Geometry check sheet. Reference: the model listing, model coordinates, mm. Face numbers are marked on the shaded views. Give positions to 0.01 mm unless a question says otherwise; leave off trailing zeros. Order: outer loops, then holes, each group sorted by start corner. A loop starts at its lowest first (then second) coordinate and runs counter-clockwise, first axis right, second up.
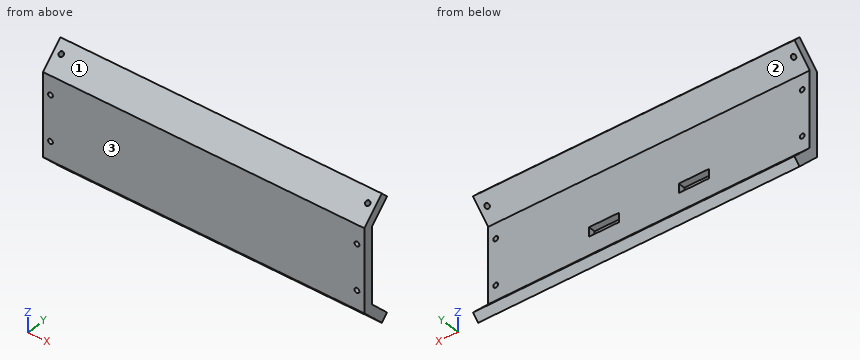
from build123d import *

# Parameters (mm, degrees)
MAIN_DEPTH                      = 107.5
F_4_0MM_DOWEL_HOLE2_D           = 3.2
F_4_0MM_DOWEL_HOLE2_ON_FACE_2_D = 3.2
F_4_0MM_DOWEL_HOLE2_ON_FACE_3_D = 3.2
F_4_0MM_DOWEL_HOLE2_ON_FACE_4_D = 3.2
SKETCH6_W                       = 20.125
SKETCH6_H                       = 6.125
SHELF_CUT_DEPTH                 = 116.995465651
SKETCH7_W                       = 20.125
SKETCH7_H                       = 6.125
BOSS_EXTRUDE2_DEPTH             = 1.4


with BuildPart() as part:
    # Sketch2 → Main (new, symmetric)
    with BuildSketch(Plane(origin=(0, 0, 0), x_dir=(0, 0, -1), z_dir=(1, 0, 0))):
        Polygon((-25, 0), (25, 0), (37.5, 12.5), (41.742640687, 8.257359313), (27.485281374, -6), (-27.485281374, -6), (-41.742640687, 8.257359313), (-37.5, 12.5), align=None)
    extrude(amount=MAIN_DEPTH, both=True)

    # Ø4.0mm Dowel Hole2 (through all)
    with Locations(Plane(origin=(-102.5, 7.071067812, -32.071067812), x_dir=(0, 0.707106781187, -0.707106781187), z_dir=(0, 0.707106781187, 0.707106781187))):
        with Locations((0, 0)):
            Hole(F_4_0MM_DOWEL_HOLE2_D / 2)

    # Ø4.0mm Dowel Hole2 on face 2 (through all)
    with Locations(Plane(origin=(-102.5, 0, -15), x_dir=(0, 0, 1), z_dir=(0, 1, 0))):
        with Locations((0, 0), (30, 0), (30, 205), (0, 205)):
            Hole(F_4_0MM_DOWEL_HOLE2_ON_FACE_2_D / 2)

    # Ø4.0mm Dowel Hole2 on face 3 (through all)
    with Locations(Plane(origin=(-102.5, 7.071067812, 32.071067812), x_dir=(0, -0.707106781187, -0.707106781187), z_dir=(0, 0.707106781187, -0.707106781187))):
        with Locations((0, 0), (0, -205)):
            Hole(F_4_0MM_DOWEL_HOLE2_ON_FACE_3_D / 2)

    # Ø4.0mm Dowel Hole2 on face 4 (through all)
    with Locations(Plane(origin=(102.5, 7.071067812, -32.071067812), x_dir=(0, 0.707106781187, -0.707106781187), z_dir=(0, 0.707106781187, 0.707106781187))):
        with Locations((0, 0)):
            Hole(F_4_0MM_DOWEL_HOLE2_ON_FACE_4_D / 2)

    # Sketch6 → Shelf cut (cut, through all)
    with BuildSketch(Plane(origin=(0, 0, 0), x_dir=(1, 0, 0), z_dir=(0, 1, 0))):
        with Locations((30, 10)):
            Rectangle(SKETCH6_W, SKETCH6_H)
        with Locations((-30, 10)):
            Rectangle(SKETCH6_W, SKETCH6_H)
    extrude(amount=-SHELF_CUT_DEPTH, mode=Mode.SUBTRACT)

    # Sketch7 → Boss-Extrude2 (add)
    with BuildSketch(Plane.XZ.offset(6)):
        with Locations((30, -10)):
            Rectangle(SKETCH7_W, SKETCH7_H)
        with Locations((-30, -10)):
            Rectangle(SKETCH7_W, SKETCH7_H)
    extrude(amount=-BOSS_EXTRUDE2_DEPTH)


solid = part.part
Item 1: Gauge pin test, flat ends, axial feed: pin 1 (5 mm diameter, centred on x = 28.5, y = -3.5, fed in from -Z); pin 2 (1.5 mm diameter, centred on x = 39, y = 6, fed in from +Z); pin 3 (1.4 mm diameter, centred on x = -30, y = -3, fed in from -Z); pin 4 (3 mm diameter, centred on x = -102.5, z = -15, fed in from +Y). Record the tip position at first contact, or that the pin passes through.
Reported:
pin 1: stops at z = -32.49
pin 2: stops at z = 40.24
pin 3: stops at z = -31.19
pin 4: passes through
Item 2: Draft check along Z on the marked faces 1, 2 and 3. Enter one of: released by +Z, released by -Z, zero draft, split by the parting line, or undercut.
Reported:
face 1: released by +Z
face 2: undercut
face 3: zero draft
Item 3: Sectioned sample at A-A (x = 38). Enter the section's corners in (y, z).
Reported:
outline: (-6, -27.49) - (8.26, -41.74) - (12.5, -37.5) - (0, -25) - (0, -13.06) - (-4.6, -13.06) - (-4.6, -6.94) - (0, -6.94) - (0, 25) - (12.5, 37.5) - (8.26, 41.74) - (-6, 27.49) - close
Item 4: Scan lines: L1, parallel to X at y = -4.8, z = 15; L2, parallel to Z at x = -102.5, y = -2.6; L3, parallel to Z at x = 102.5, y = -1.9. Record each from-to range of solid material in increasing order.
Reported:
L1: x = -107.5 to -104.1, -100.9 to 100.9, 104.1 to 107.5
L2: z = -30.89 to -16.6, -13.4 to 13.4, 16.6 to 30.89
L3: z = -31.59 to -16.6, -13.4 to 13.4, 16.6 to 31.59
Item 5: Sectioned sample at B-B (y = -2). Enter the section's corners in (x, z).
Reported:
outline: (-107.5, -31.49) - (107.5, -31.49) - (107.5, 31.49) - (-107.5, 31.49) - close; hole circle Ø3.2 at (-102.5, -15); hole circle Ø3.2 at (-102.5, 15); hole (-40.06, -13.06) - (-19.94, -13.06) - (-19.94, -6.94) - (-40.06, -6.94) - close; hole (19.94, -13.06) - (40.06, -13.06) - (40.06, -6.94) - (19.94, -6.94) - close; hole circle Ø3.2 at (102.5, -15); hole circle Ø3.2 at (102.5, 15)
Item 6: Sectioned sample at C-C (x = -63.5). Enter the section's corners in (y, z).
Reported:
outline: (-6, -27.49) - (8.26, -41.74) - (12.5, -37.5) - (0, -25) - (0, 25) - (12.5, 37.5) - (8.26, 41.74) - (-6, 27.49) - close
